from build123d import *

# Parameters (mm, degrees)
F0_R     = 3.2639
F0_R_2   = 2.5527
F1_DEPTH = 6.35


with BuildPart() as f1:
    # F0 (on Front) → F1 (new body)
    with BuildSketch(Plane.XZ):
        with BuildLine():
            Line((175.26, 0), (2.54, 0))
            ThreePointArc((2.54, 0), (0.743949, -0.743949), (0, -2.54))
            Line((0, -2.54), (0, -25.04426))
            ThreePointArc((0, -25.04426), (0.024551, -25.396562), (0.097729, -25.742052))
            Line((0.097729, -25.742052), (50.273655, -201.357792))
            ThreePointArc((50.273655, -201.357792), (51.186349, -202.687806), (52.715926, -203.2))
            Line((52.715926, -203.2), (125.084074, -203.2))
            ThreePointArc((125.084074, -203.2), (126.613651, -202.687806), (127.526345, -201.357792))
            Line((127.526345, -201.357792), (177.702271, -25.742052))
            ThreePointArc((177.702271, -25.742052), (177.775449, -25.396562), (177.8, -25.04426))
            Line((177.8, -25.04426), (177.8, -2.54))
            ThreePointArc((177.8, -2.54), (177.056051, -0.743949), (175.26, 0))
        make_face()
        with Locations((69.85, -196.85)):
            Circle(F0_R, mode=Mode.SUBTRACT)
        with Locations((107.95, -196.85)):
            Circle(F0_R, mode=Mode.SUBTRACT)
        with Locations((69.85, -88.9)):
            Circle(F0_R, mode=Mode.SUBTRACT)
        with Locations((12.7, -6.35)):
            Circle(F0_R_2, mode=Mode.SUBTRACT)
        with Locations((107.95, -88.9)):
            Circle(F0_R, mode=Mode.SUBTRACT)
        with Locations((165.1, -6.35)):
            Circle(F0_R_2, mode=Mode.SUBTRACT)
    extrude(amount=F1_DEPTH)


solid = f1.part
Can you work these out from the model? Positions are in its coordinate system, mm. Coordinates: 2 decimals unless noted, no trailing zeros. Write each loop counter-clockwise with the first axis right and the second up, starting at its lowest first coordinate (ties: lowest second). Pieces come first, ordered by that corner, then holes. Notation, with made-up numbers: M -20.75,-14.75 L 6.25,-14.75 A25 cw 6.25,13.25 Z; hole C -34.5,48.5 d11. An arc over 180 degrees is marked long. Use one line per item in the form item = value.
Q1. If we section it at B-B (y = -5): Write out the boundary of the cut face in (x, z).
Model answer:
outline = M 0,-25.04 A2.54 ccw 0.1,-25.74 L 50.27,-201.36 A2.54 ccw 52.72,-203.2 L 125.08,-203.2 A2.54 ccw 127.53,-201.36 L 177.7,-25.74 A2.54 ccw 177.8,-25.04 L 177.8,-2.54 A2.54 ccw 175.26,0 L 2.54,0 A2.54 ccw 0,-2.54 Z; hole C 12.7,-6.35 d5.11; hole C 69.85,-196.85 d6.53; hole C 69.85,-88.9 d6.53; hole C 107.95,-196.85 d6.53; hole C 107.95,-88.9 d6.53; hole C 165.1,-6.35 d5.11
Q2. If we section it at C-C (z = -6.35): Write out the boundary of the cut face in (x, y).
Model answer:
outline = M 0,-6.35 L 10.15,-6.35 L 10.15,0 L 0,0 Z; M 15.25,-6.35 L 162.55,-6.35 L 162.55,0 L 15.25,0 Z; M 167.65,-6.35 L 177.8,-6.35 L 177.8,0 L 167.65,0 Z
Q3. If we section it at D-D (x = 107.95): Write out the boundary of the cut face in (y, z), then the cut area to 3 significant figures.
Model answer:
outline = M -6.35,-203.2 L 0,-203.2 L 0,-200.11 L -6.35,-200.11 Z; M -6.35,-193.59 L 0,-193.59 L 0,-92.16 L -6.35,-92.16 Z; M -6.35,-85.64 L 0,-85.64 L 0,0 L -6.35,0 Z
area = 1,210 mm^2
Q4. For P1, Ø4.5, axis at x = 12.7, z = -6.35, coming from the +Y side; P2, Ø1, axis at y = -3.5, z = -142, coming from the -X side, each with a flat end and sliding along its axis, tell me the tip position at first contact or that it passes through.
Model answer:
P1 = through
P2 = 33.17
Q5. If we section it at A-A (x = 165.1): Write out the boundary of the cut face in (y, z), then the cut area to 3 significant figures.
Model answer:
outline = M -6.35,-69.85 L 0,-69.85 L 0,-8.9 L -6.35,-8.9 Z; M -6.35,-3.8 L 0,-3.8 L 0,0 L -6.35,0 Z
area = 411 mm^2
Q6. We'd pull the mould along Z, two halves only. Please class faces 1 (the cylindrical face through (167.535, -3.131, -5.583)), 2 (the flat face through (90, -3, 0)), 3 (the cylindrical face through (15.135, -3.131, -5.583)), 4 (the flat face through (177.8, -3, -14)): +Z half, -Z half, draft (parallel to the pull), parting line (faces both ways), or undercut.
Model answer:
face_1 = undercut
face_2 = +Z half
face_3 = undercut
face_4 = draft
Q7. I need wall thicknesses on line 1 along Z through (x, y) = (69.85, -1.5); line 2 along X through (y, z) = (-5, -196.85); line 3 along X through (y, z) = (-5, -97.5). Which ranges of each line are inside material? Lowest first, please. Write a range as from..to.
Model answer:
line_1 = -203.2..-200.11, -193.59..-92.16, -85.64..0
line_2 = 48.99..66.59, 73.11..104.69, 111.21..128.81
line_3 = 20.6..157.2
